Input: part model. Units: mm. Frame: model coordinates. A direction names the side the tool comes from. Coordinates: 2 decimals unless noted, no trailing zeros. Loops run counter-clockwise (first coordinate to the right, second up) from the corner with the lowest first, then second, coordinate; pieces in that order, holes last.
```python
from build123d import *

# Parameters (mm, degrees)
SKETCH1_W           = 8
SKETCH1_H           = 12
SKETCH1_R           = 2.5
BOSS_EXTRUDE1_DEPTH = 5.08
SKETCH2_W           = 4
SKETCH2_H           = 3
BOSS_EXTRUDE2_DEPTH = 5.08


with BuildPart() as part:
    # Sketch1 → Boss-Extrude1 (new body)
    with BuildSketch(Plane(origin=(0, 0, 0), x_dir=(1, 0, 0), z_dir=(0, 1, 0))):
        with Locations((0, -2)):
            Rectangle(SKETCH1_W, SKETCH1_H)
        Circle(SKETCH1_R, mode=Mode.SUBTRACT)
    extrude(amount=BOSS_EXTRUDE1_DEPTH)

    # Sketch2 → Boss-Extrude2 (add)
    with BuildSketch(Plane(origin=(0, 5.08, 0), x_dir=(1, 0, 0), z_dir=(0, 1, 0))):
        with Locations((6, -6.5)):
            Rectangle(SKETCH2_W, SKETCH2_H)
        Polygon((-4, -8), (-4, -16.08), (8, -16.08), (8, -13.08), (4, -13.08), (4, -8), align=None)
    extrude(amount=-BOSS_EXTRUDE2_DEPTH)


solid = part.part
```
Item 1: Section query B-B (z = 0). Output: boundary loops of the cut face in (x, y).
Result:
outline: (-4, 0) - (-2.5, 0) - (-2.5, 5.08) - (-4, 5.08) - close; (2.5, 0) - (4, 0) - (4, 5.08) - (2.5, 5.08) - close
Item 2: Section query C-C (y = 2). Output: boundary loops of the cut face in (x, z), then the cut area to 3 significant figures.
Result:
outline: (-4, -4) - (4, -4) - (4, 5) - (8, 5) - (8, 8) - (4, 8) - (4, 13.08) - (8, 13.08) - (8, 16.08) - (-4, 16.08) - close; hole circle Ø5 at (0, 0)
area: 165 mm2
Item 3: Section query D-D (z = 8.5). Output: boundary loops of the cut face in (x, y), then the cut area to 3 significant figures.
Result:
outline: (-4, 0) - (4, 0) - (4, 5.08) - (-4, 5.08) - close
area: 40.6 mm2
Item 4: Line query: L1, parallel to X at y = 1.6, z = 0; L2, parallel to Z at x = 0, y = 2.8; L3, parallel to X at y = 2.3, z = 8.25. Output: solid intervals per line, ascending.
Result:
L1: x = -4 to -2.5, 2.5 to 4
L2: z = -4 to -2.5, 2.5 to 16.08
L3: x = -4 to 4
Item 5: Reachability of faces 1 (the face through (4, 3, 1)), 2 (the face through (6, 3, 13.08)), 3 (the face through (1, 0, 8)) from +Z, -Z, +X, -X, +Y, -Y: full face, straight path, thin tool, end or side. Return the list, or none.
Result:
face 1: -Z, +X, +Y, -Y
face 2: +X, +Y, -Y
face 3: +Z, -Z, +X, -X, -Y
Item 6: Mould query, pull axis X, two halves, no side actions, for faces 4 (the face through (8, 3, 15)), 5 (the face through (-0.54, 2.5, 2.44)), 6 (the face through (1, 5.08, 8)), 7 (the face through (-4, 3, 6)). Classes: +X half, -X half, draft (parallel to the pull), parting line (faces both ways), or undercut.
Result:
face 4: +X half
face 5: undercut
face 6: draft
face 7: -X half
Item 7: Section query A-A (x = 4.5). Output: boundary loops of the cut face in (y, z).
Result:
outline: (0, 5) - (5.08, 5) - (5.08, 8) - (0, 8) - close; (0, 13.08) - (5.08, 13.08) - (5.08, 16.08) - (0, 16.08) - close
Item 8: Contact query for flat-ended pins moving along their axis: P1, Ø3, axis at x = 6, y = 2, coming from the -Z side; P2, Ø1.5, axis at y = 2, z = -1.5, coming from the +X side. Output: stop coordinate, or through.
Result:
P1: stops at z = 5
P2: stops at x = 4
